CAD build for the part. Positions are in the model's coordinates, mm. Face numbers are marked on the shaded views. A direction names the side the tool comes from. Give positions to 0.01 mm unless a question says otherwise; leave off trailing zeros. Write each loop counter-clockwise with the first axis right and the second up, starting at its lowest first coordinate (ties: lowest second). Pieces come first, ordered by that corner, then holes. Notation, with made-up numbers: (-32, 77.5) - (-17, 77.5) arc R20 cw to (-17, 97.5) - close; hole circle Ø1 at (2, 39). An arc over 180 degrees is marked (long way). Put each result on its own line as item: value. Start each with the question number.
1. Tool access for the marked faces 1, 2 and 3: list every direction of +Z, -Z, +X, -X, +Y, -Y with a clear straight run to the whole face (end or side of a thin tool).
2. Cut at B-B on z = -16. List the corners of the cut face in (x, y), and give its area (3 significant figures).
3. Mould opens along X. For the marked faces 4, 5, 6 and 7 say: +X half, -X half, draft (parallel to the pull), parting line (faces both ways), or undercut.
4. Drop flat-ended pins along their axis: pin 1 (3.5 mm diameter, centred on x = 15, z = -5, fed in from +Y); pin 2 (2.5 mm diameter, centred on x = -1, y = 31, fed in from -Z); pin 3 (2.5 mm diameter, centred on x = 57, y = 1, fed in from -Z). Give the stop position or say it passes through.
5. Cut at C-C on x = 32. List the corners of the cut face in (y, z).
6. Wall check: line 1 (Z direction, x = 103, y = 1.3); line 2 (X direction, y = 2.1, z = -35); line 3 (X direction, y = 11, z = -10). Give the ranges that are in metal, low to high.
7. Cut at A-A on x = 15. List the corners of the cut face in (y, z), and give its area (3 significant figures).
from build123d import *

# Parameters (mm, degrees)
SKETCH_1_W          = 20
SKETCH_1_H          = 38
SKETCH_1_R          = 1.6
EXTRUDE_1_DEPTH     = 3
SKETCH_7_W          = 38
SKETCH_7_H          = 3
EXTRUDE_7_DEPTH     = 6
EXTRUDE_8_DEPTH     = 19
FILLET_1_R          = 2
SKETCH_10_R         = 1.6
CUT_EXTRUDE_3_DEPTH = 10
CUT_EXTRUDE_4_DEPTH = 3
SKETCH_13_W         = 10
SKETCH_13_H         = 46.172897719
CUT_EXTRUDE_5_DEPTH = 3
FILLET_3_R          = 10
FILLET_4_R          = 5
FILLET_5_R          = 2
FILLET_6_R          = 5
FILLET_7_R          = 5
FILLET_8_R          = 3
SKETCH_11_W         = 39
SKETCH_11_H         = 38
EXTRUDE_9_DEPTH     = 3
FILLET_START        = -37.531780157
FILLET_9_DEPTH      = 9.135274029
FILLET_START_2      = -9
FILLET_9_2_DEPTH    = 9
FILLET_START_3      = -38.0000001
FILLET_9_3_DEPTH    = 14.603493972
FILLET_START_4      = -14
FILLET_9_4_DEPTH    = 5
FILLET_9_5_DEPTH    = 5


with BuildPart() as part:
    # 草图1 → 凸台-拉伸1 (new body)
    with BuildSketch(Plane(origin=(0, 0, 0), x_dir=(1, 0, 0), z_dir=(0, 1, 0))):
        with Locations((10, 19)):
            Rectangle(SKETCH_1_W, SKETCH_1_H)
        with Locations(Location((15, 5, 0), (0, 0, 270))):
            Circle(SKETCH_1_R, mode=Mode.SUBTRACT)
        with Locations(Location((15, 35, 0), (0, 0, 270))):
            Circle(SKETCH_1_R, mode=Mode.SUBTRACT)
    extrude(amount=EXTRUDE_1_DEPTH)

    # 草图7 → 凸台-拉伸7 (add)
    with BuildSketch(Plane.ZY):
        with BuildLine():
            Line((-38, 3), (0, 3))
            Line((0, 3), (0, 60))
            Line((0, 60), (-38, 60))
            add(Edge.make_bspline(
                [(-38, 3), (-35.160021148, 31.761534368), (-38, 60)],
                knots=[0, 0, 0, 0.545624852, 0.545624852, 0.545624852], degree=2))
        make_face()
        with Locations((-19, 1.5)):
            Rectangle(SKETCH_7_W, SKETCH_7_H)
        with BuildLine():
            Line((-38, 60), (0, 60))
            Line((0, 60), (2.121320344, 62.121320344))
            Line((2.121320344, 62.121320344), (-44.669984364, 108.912625051))
            Line((-44.669984364, 108.912625051), (-46.669047558, 106.669047558))
            add(Edge.make_bspline(
                [(-38, 60), (-40.365023894, 83.51589552), (-46.669047558, 106.669047558)],
                knots=[0.545624852, 0.545624852, 0.545624852, 1, 1, 1], degree=2))
        make_face()
    extrude(amount=EXTRUDE_7_DEPTH)

    # 草图8 → 凸台-拉伸8 (add)
    with BuildSketch(Plane.ZY.offset(6)):
        Polygon((-44.669984364, 108.912625051), (-46.669047558, 106.669047558), (0, 60), (2.121320344, 62.121320344), align=None)
    extrude(amount=-EXTRUDE_8_DEPTH)

    # 圆角1
    fillet_1_edges = [part.edges().sort_by_distance(p)[0] for p in [
        (-3, 60, 0),
    ]]
    fillet(fillet_1_edges, radius=FILLET_1_R)

    # 草图10 → 切除-拉伸3 (cut)
    with BuildSketch(Plane(origin=(0, 32.121320344, 32.121320344), x_dir=(1, 0, 0), z_dir=(0, 0.7071067811865476, 0.7071067811865475))):
        with Locations(Location((8, 102.866406871, 0), (0, 0, 270))):
            Circle(SKETCH_10_R)
        with Locations(Location((8, 47.986406871, 0), (0, 0, 270))):
            Circle(SKETCH_10_R)
    extrude(amount=-CUT_EXTRUDE_3_DEPTH, mode=Mode.SUBTRACT)

    # 草图12 → 切除-拉伸4 (cut)
    with BuildSketch(Plane(origin=(0, 0, 0), x_dir=(0, 0, -1), z_dir=(1, 0, 0))):
        with BuildLine():
            Line((9, 57), (9, 3))
            Line((9, 3), (29, 3))
            add(Edge.make_bspline(
                [(29, 3), (25.530992691, 30.329804849), (29, 57)],
                knots=[0, 0, 0, 0.681816387, 0.681816387, 0.681816387], degree=2))
            Line((29, 57), (9, 57))
        make_face()
        with BuildLine():
            Line((33.748737342, 81.748737342), (9, 57))
            Line((9, 57), (29, 57))
            add(Edge.make_bspline(
                [(29, 57), (30.618883469, 69.446194026), (33.748737342, 81.748737342)],
                knots=[0.681816387, 0.681816387, 0.681816387, 1, 1, 1], degree=2))
        make_face()
    extrude(amount=-CUT_EXTRUDE_4_DEPTH, mode=Mode.SUBTRACT)

    # 草图13 → 切除-拉伸5 (cut)
    with BuildSketch(Plane(origin=(0, 32.121320344, 32.121320344), x_dir=(1, 0, 0), z_dir=(0, 0.7071067811865476, 0.7071067811865475))):
        with Locations((8, 75.512855731)):
            Rectangle(SKETCH_13_W, SKETCH_13_H)
    extrude(amount=-CUT_EXTRUDE_5_DEPTH, mode=Mode.SUBTRACT)

    # 圆角3
    fillet_3_edges = [part.edges().sort_by_distance(p)[0] for p in [
        (-1.5, 57, -9),
    ]]
    fillet(fillet_3_edges, radius=FILLET_3_R)

    # 圆角4
    fillet_4_edges = [part.edges().sort_by_distance(p)[0] for p in [
        (-1.5, 3, -29),
        (-1.5, 3, -9),
    ]]
    fillet(fillet_4_edges, radius=FILLET_4_R)

    # 圆角5
    fillet_5_edges = [part.edges().sort_by_distance(p)[0] for p in [
        (-1.5, 81.748737342, -33.748737342),
    ]]
    fillet(fillet_5_edges, radius=FILLET_5_R)

    # 圆角6
    fillet_6_edges = [part.edges().sort_by_distance(p)[0] for p in [
        (3, 100.780897067, -38.659576724),
    ]]
    fillet(fillet_6_edges, radius=FILLET_6_R)

    # 圆角7
    fillet_7_edges = [part.edges().sort_by_distance(p)[0] for p in [
        (3, 68.131727984, -6.01040764),
    ]]
    fillet(fillet_7_edges, radius=FILLET_7_R)

    # 圆角8
    fillet_8_edges = [part.edges().sort_by_distance(p)[0] for p in [
        (13, 61.060660172, 1.060660172),
        (13, 107.790836305, -45.669515961),
        (13, 100.780897067, -38.659576724),
        (13, 68.131727984, -6.01040764),
    ]]
    fillet(fillet_8_edges, radius=FILLET_8_R)

    # 草图11 → 凸台-拉伸9 (add)
    with BuildSketch(Plane(origin=(0, 0, 0), x_dir=(1, 0, 0), z_dir=(0, 1, 0))):
        with Locations((39.5, 19)):
            Rectangle(SKETCH_11_W, SKETCH_11_H)
    extrude(amount=EXTRUDE_9_DEPTH)

    # 圆角9: read off the stored shape, not the designer's step
    # 圆角9 outline → 圆角9 (add)
    with BuildSketch(Plane.XY.offset(FILLET_START)):
        with BuildLine():
            Line((0, 3), (5, 3))
            ThreePointArc((5, 3), (1.464466094, 4.464466094), (0, 8))
            Line((0, 8), (0, 3))
        make_face()
    extrude(amount=FILLET_9_DEPTH)

    # Fillet 9 2 outline → Fillet 9 2 (add)
    with BuildSketch(Plane.XY.offset(FILLET_START_2)):
        with BuildLine():
            Line((0, 3), (5, 3))
            ThreePointArc((5, 3), (1.464466094, 4.464466094), (0, 8))
            Line((0, 8), (0, 3))
        make_face()
    extrude(amount=FILLET_9_2_DEPTH)

    # Fillet 9 3 outline → Fillet 9 3 (add)
    with BuildSketch(Plane.XY.offset(FILLET_START_3)):
        with BuildLine():
            Line((0, 3), (5, 3))
            ThreePointArc((5, 3), (1.464466094, 4.464466094), (0, 8))
            Line((0, 8), (0, 3))
        make_face()
    extrude(amount=FILLET_9_3_DEPTH)

    # Fillet 9 4 outline → Fillet 9 4 (add)
    with BuildSketch(Plane.XY.offset(FILLET_START_4)):
        with BuildLine():
            Line((0, 3), (5, 3))
            ThreePointArc((5, 3), (1.464466094, 4.464466094), (0, 8))
            Line((0, 8), (0, 3))
        make_face()
    extrude(amount=FILLET_9_4_DEPTH)

    # Fillet 9 5 outline → Fillet 9 5 (cut)
    with BuildSketch(Plane.YZ):
        with BuildLine():
            Line((3, -14), (8, -14))
            Line((8, -14), (8, -9))
            ThreePointArc((8, -9), (4.464466094, -10.464466094), (3, -14))
        make_face()
        with BuildLine():
            Line((8, -38.0000001), (8, -37.548880036))
            add(Edge.make_bspline(
                [(3, -38), (5.50197912, -37.752948932), (8, -37.548880036)],
                knots=[0, 0, 0, 0.047464157, 0.047464157, 0.047464157], degree=2))
            Line((3, -38), (8, -38.0000001))
        make_face()
        with BuildLine():
            ThreePointArc((3, -23.396506128), (4.464466094, -26.932040034), (8, -28.396506128))
            Line((8, -28.396506128), (8, -23.396506128))
            Line((8, -23.396506128), (3, -23.396506128))
        make_face()
    extrude(amount=FILLET_9_5_DEPTH, mode=Mode.SUBTRACT)

    # 镜向6: part across plane


with BuildPart() as part_1:
    add(part.part)
    add(part.part.mirror(Plane(origin=(59, 0, 0), x_dir=(0, 0, 1), z_dir=(1, 0, 0))))


solid = part_1.part
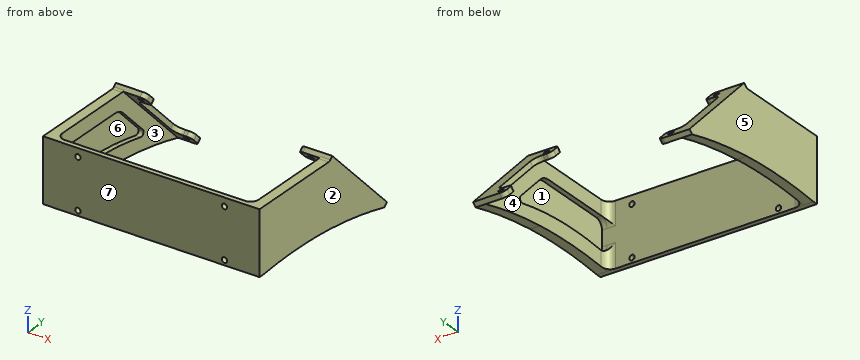
Report:
1. face 1: none
1. face 2: +Z, -Z, +X, +Y, -Y
1. face 3: -Z
2. outline: (-6, 0) - (124, 0) - (124, 80.24) - (115, 80.24) - (115, 76) - (118, 76) - (118, 64) - (121, 64) - (121, 3) - (-3, 3) - (-3, 64) - (0, 64) - (0, 76) - (3, 76) - (3, 80.24) - (-6, 80.24) - close
2. area: 976 mm²
3. face 4: undercut
3. face 5: -X half
3. face 6: undercut
3. face 7: draft
4. pin 1: stops at y = 3
4. pin 2: stops at z = -36.59
4. pin 3: stops at z = -38
5. outline: (0, -38) - (3, -38) - (3, 0) - (0, 0) - close
6. line 1: z = -38 to -36.6, -33.4 to -6.6, -3.4 to 0
6. line 2: x = -6 to 13.4, 16.6 to 101.4, 104.6 to 124
6. line 3: x = -6 to -3, 121 to 124
7. outline: (0, -38) - (3, -38) - (3, -36.6) - (0, -36.6) - close; (0, -33.4) - (3, -33.4) - (3, -6.6) - (0, -6.6) - close; (0, -3.4) - (3, -3.4) - (3, 0) - (0, 0) - close
7. area: 94.8 mm²
